```python
from build123d import *

# Parameters (mm, degrees)
BOSS_EXTRUDE1_DEPTH = 119.376
SKETCH2_R           = 6
CUT_EXTRUDE1_DEPTH  = 56
SKETCH3_R           = 6
CUT_EXTRUDE2_DEPTH  = 56


with BuildPart() as part:
    # Sketch1 → Boss-Extrude1 (new body)
    with BuildSketch(Plane(origin=(0, 0, 0), x_dir=(1, 0, 0), z_dir=(0, 1, 0))):
        with BuildLine():
            Line((0, -32.5), (0, 32.5))
            ThreePointArc((0, 32.5), (-32.5, 0), (0, -32.5))
        make_face()
    extrude(amount=-BOSS_EXTRUDE1_DEPTH)

    # Sketch2 → Cut-Extrude1 (cut)
    with BuildSketch(Plane(origin=(0, 0, 0), x_dir=(0, 0, -1), z_dir=(1, 0, 0))):
        with Locations((0, -15.894)):
            Circle(SKETCH2_R)
    extrude(amount=-CUT_EXTRUDE1_DEPTH, mode=Mode.SUBTRACT)

    # Sketch3 → Cut-Extrude2 (cut)
    with BuildSketch(Plane(origin=(0, 0, 0), x_dir=(0, 0, -1), z_dir=(1, 0, 0))):
        with Locations((0, -101.376)):
            Circle(SKETCH3_R)
    extrude(amount=-CUT_EXTRUDE2_DEPTH, mode=Mode.SUBTRACT)


solid = part.part
```
Design review of the part built by this model. Coordinates are the model's own, in mm. Coordinates: 2 decimals unless noted, no trailing zeros. Order: outer loops, then holes, each group sorted by start corner. A loop starts at its lowest first (then second) coordinate and runs counter-clockwise, first axis right, second up. Notation, with made-up numbers: (-24, 8) - (5, 8) arc R19 cw to (5, 42) - close; hole circle Ø7 at (37, 68). An arc over 180 degrees is marked (long way). One line per question, with ' | ' between items.
Q1. Consider section B-B, the plane y = -30. Give the boundary of the cut face in (x, z), then the cut area to 3 significant figures.
Answer key:
outline: (0, -32.5) - (0, 32.5) arc R32.5 ccw to start | area: 1,660 mm2
Q2. Clearance check with flat-ended pins moving along their axes: pin 1 Ø6 at (x, y) = (-15.5, -65.5) entering from -Z; pin 2 Ø10 at (y, z) = (-101.5, -13.5) entering from -X; pin 3 Ø1 at (x, y) = (-27.5, -60.5) entering from +Z. State where each tip first meets the part, or that it passes through.
Answer key:
pin 1: stops at z = -30 | pin 2: stops at x = -31.37 | pin 3: stops at z = 18.09
Q3. Consider section D-D, the plane x = -20. Give the boundary of the cut face in (y, z).
Answer key:
outline: (-119.38, -25.62) - (0, -25.62) - (0, 25.62) - (-119.38, 25.62) - close; hole circle Ø12 at (-101.38, 0); hole circle Ø12 at (-15.89, 0)
Q4. The part is to be moulded in two halves that separate along Y. For faces 1 (the flat face through (-13, -119.376, 0)), 2 (the cylindrical face through (-16, -16, 6)), 3 (the flat face through (0, -59, 0)), say which applies: +Y half, -Y half, draft (parallel to the pull), parting line (faces both ways), or undercut.
Answer key:
face 1: -Y half | face 2: undercut | face 3: draft
Q5. To check wall thickness, follow line 1 along Y through (x, z) = (-9, 0); line 2 along Y through (x, z) = (-14, -4); line 3 along X through (y, z) = (-64.5, 15). State the ranges of each line that lie inside material, in increasing order.
Answer key:
line 1: y = -119.38 to -107.38, -95.38 to -21.89, -9.89 to 0 | line 2: y = -119.38 to -105.85, -96.9 to -20.37, -11.42 to 0 | line 3: x = -28.83 to 0
Q6. Consider section C-C, the plane z = 8. Give the boundary of the cut face in (x, y).
Answer key:
outline: (-31.5, -119.38) - (0, -119.38) - (0, 0) - (-31.5, 0) - close
Q7. Consider section A-A, the plane z = 0. Give the boundary of the cut face in (x, y), then the cut area to 3 significant figures.
Answer key:
outline: (-32.5, -119.38) - (0, -119.38) - (0, -107.38) - (-32.5, -107.38) - close; (-32.5, -95.38) - (0, -95.38) - (0, -21.89) - (-32.5, -21.89) - close; (-32.5, -9.89) - (0, -9.89) - (0, 0) - (-32.5, 0) - close | area: 3,100 mm2
